```python
from build123d import *

# Parameters (mm, degrees)
BOSS_EXTRUDE1_DEPTH = 10
SKETCH2_R           = 7
BOSS_EXTRUDE2_DEPTH = 6


with BuildPart() as part:
    # Sketch1 → Boss-Extrude1 (new body)
    with BuildSketch(Plane.XY):
        with BuildLine():
            ThreePointArc((-43.08998785, 39.062645298), (50.557727896, 22.443015988), (126.455624698, -34.877277135))
            ThreePointArc((126.455624698, -34.877277135), (140.904450524, -64.085787948), (108.507084419, -60.576323444))
            ThreePointArc((108.507084419, -60.576323444), (40.525240485, -8.589143953), (-43.08998785, 9.650689563))
            ThreePointArc((-43.08998785, 9.650689563), (-83.811407941, 24.356667431), (-43.08998785, 39.062645298))
        make_face()
    extrude(amount=BOSS_EXTRUDE1_DEPTH)

    # Sketch2 → Boss-Extrude2 (add)
    with BuildSketch(Plane.XY.offset(10)):
        with Locations((125.668384571, -53.444726012)):
            Circle(SKETCH2_R)
        with Locations((-60.795267601, 24.356667431)):
            Circle(SKETCH2_R)
    extrude(amount=BOSS_EXTRUDE2_DEPTH)


solid = part.part
```
Model file for the job. Use its own axes, mm. A direction names the side the tool comes from. Coordinates: 2 decimals unless noted, no trailing zeros. Order: outer loops, then holes, each group sorted by start corner. A loop starts at its lowest first (then second) coordinate and runs counter-clockwise, first axis right, second up. Notation, with made-up numbers: (26.5, 7.25) - (63.5, 7.25) arc R23 ccw to (63.5, 26.25) - close; hole circle Ø2 at (68, -27). An arc over 180 degrees is marked (long way). Return JSON: item names as keys, results as strings. Group by question number.
1) Saw through at B-B, the plane y = -58. Write the cut outline in (x, z), plus the area to 3 significant figures.
2) Saw through at D-D, the plane z = 4.75. Write the cut outline in (x, y).
3) Probe line 1 (Z direction, x = 9, y = 27); line 2 (Y direction, x = 19, z = 5.5); line 3 (Y direction, x = 91, z = 2). List the from-to ranges inside material, lowest first. Write a range as from..to.
4) Flat gauge pins, fed straight in: P1, Ø2, axis at x = 21, y = 25.5, coming from the +Z side; P2, Ø1, axis at y = -10, z = 5, coming from the -X side. Where does each tip first touch, or does it go through?
5) Mould opens along X. For faces 1 (the flat face through (31, -3, 10)), 2 (the cylindrical face through (141.216, -63.625, 4.93)), 3 (the cylindrical face through (41.62, -9.1, 4.93)) say: released by +X, released by -X, zero draft, split by the parting line, or undercut.
6) Saw through at A-A, the plane y = 3.5. Write the cut outline in (x, z), plus the area to 3 significant figures.
7) Saw through at C-C, the plane x = 52.5. Write the cut outline in (y, z), plus the area to 3 significant figures.
8) Tool access for faces 4 (the flat face through (126, -53, 16)), 5 (the cylindrical face through (132.345, -51.342, 12.958)): list every direction of +Z, -Z, +X, -X, +Y, -Y with a clear straight run to the whole face (end or side of a thin tool).
Values found:
{
 "1": {"outline": "(106.3, 0) - (143.69, 0) - (143.69, 10) - (130.98, 10) - (130.98, 16) - (120.35, 16) - (120.35, 10) - (106.3, 10) - close", "area": "438 mm²"},
 "2": {"outline": "(-43.09, 9.65) arc R196.93 cw to (108.51, -60.58) arc R18.58 ccw (long way) to (126.46, -34.88) arc R203.73 ccw to (-43.09, 39.06) arc R23.02 ccw (long way) to start"},
 "3": {"line 1": "z = 0..10", "line 2": "y = -0.12..33.23", "line 3": "y = -42.28..-1.05"},
 "4": {"P1": "stops at z = 10", "P2": "stops at x = 42.46"},
 "5": {"face 1": "zero draft", "face 2": "split by the parting line", "face 3": "undercut"},
 "6": {"outline": "(-70.53, 0) - (-51.06, 0) - (-51.06, 10) - (-70.53, 10) - close; (6.59, 0) - (84.65, 0) - (84.65, 10) - (6.59, 10) - close", "area": "975 mm²"},
 "7": {"outline": "(-14.64, 0) - (21.58, 0) - (21.58, 10) - (-14.64, 10) - close", "area": "362 mm²"},
 "8": {"face 4": "+Z, +X, -X, +Y, -Y", "face 5": "+Z"}
}
